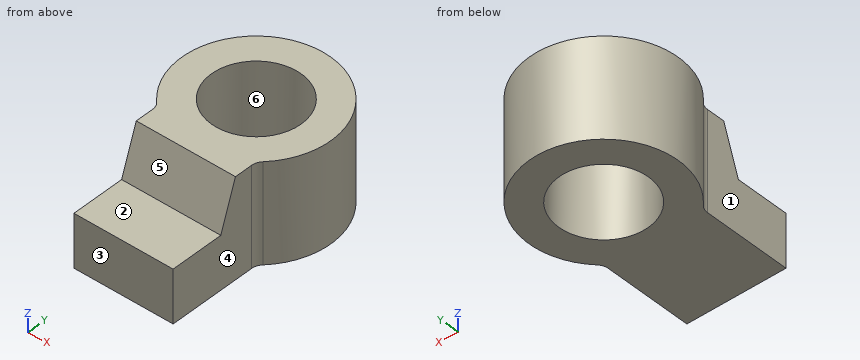
from build123d import *

# Parameters (mm, degrees)
F0_R     = 22.932499
F1_DEPTH = 50.8
F3_DEPTH = 38.1


with BuildPart() as f1:
    # F0 (on Top) → F1 (new body)
    with BuildSketch(Plane.XY):
        with BuildLine():
            ThreePointArc((25.377046, 2.454483), (25.848974, 4.856726), (27.194611, 6.901902))
            ThreePointArc((27.194611, 6.901902), (0, 71.686413), (-27.194611, 6.901902))
            ThreePointArc((-27.194611, 6.901902), (-25.848974, 4.856726), (-25.377046, 2.454483))
            Line((-25.377046, 2.454483), (-25.377046, -42.613587))
            Line((-25.377046, -42.613587), (25.377046, -42.613587))
            Line((25.377046, -42.613587), (25.377046, 2.454483))
        make_face()
        with Locations((0, 33.586413)):
            Circle(F0_R, mode=Mode.SUBTRACT)
    extrude(amount=F1_DEPTH)

    # F2 (on Right) → F3 (cut, symmetric)
    with BuildSketch(Plane.YZ):
        Polygon((-47.515366, 27.248772), (-42.938434, 27.030824), (-15.25889, 27.030824), (-4.361433, 57.761654), (-47.515366, 57.761654), align=None)
    extrude(amount=F3_DEPTH, both=True, mode=Mode.SUBTRACT)


solid = f1.part
Design review of the part built by this model. Coordinates are the model's own, in mm. Face numbers are marked on the shaded views. A direction names the side the tool comes from. Coordinates: 2 decimals unless noted, no trailing zeros. Order: outer loops, then holes, each group sorted by start corner. A loop starts at its lowest first (then second) coordinate and runs counter-clockwise, first axis right, second up. Notation, with made-up numbers: (88.5, 47.25) - (95.5, 47.25) arc R14 ccw to (95.5, 65.25) - close; hole circle Ø3 at (18.5, 30.5). An arc over 180 degrees is marked (long way). Put each result on its own line as item: value.
1) Take a section at D-D, the plane x = -21. Give the boundary of the cut face in (y, z), and give its area (3 significant figures).
Response values:
outline: (-42.61, 0) - (24.37, 0) - (24.37, 50.8) - (-6.83, 50.8) - (-15.26, 27.03) - (-42.61, 27.03) - close; (42.8, 0) - (65.38, 0) - (65.38, 50.8) - (42.8, 50.8) - close
area: 3,800 mm²
2) Take a section at A-A, the plane x = 0. Give the boundary of the cut face in (y, z), and give its area (3 significant figures).
Response values:
outline: (-42.61, 0) - (10.65, 0) - (10.65, 50.8) - (-6.83, 50.8) - (-15.26, 27.03) - (-42.61, 27.03) - close; (56.52, 0) - (71.69, 0) - (71.69, 50.8) - (56.52, 50.8) - close
area: 2,730 mm²
3) Insertion check: P1, Ø12, axis at x = 18, z = 12, coming from the +Y side; P2, Ø22, axis at x = 3, y = -33.5, coming from the +Z side; P3, Ø22.5, axis at y = -21.5, z = 30.5, coming from the +X side. Each pin has a flat end and moves straight along its axis. Give the tip position at first contact, or say it passes through.
Response values:
P1: stops at y = 69.75
P2: stops at z = 27.03
P3: stops at x = 25.38
4) Wall thickness on L1, parallel to Y at x = 0, z = 23; L2, parallel to Z at x = -25, y = -19; L3, parallel to X at y = 2.5, z = 43: over which ranges is each line inside the solid? List them lowest first. Write a range as from..to.
Response values:
L1: y = -42.61..10.65, 56.52..71.69
L2: z = 0..27.03
L3: x = -25.38..25.38
5) Take a section at B-B, the plane y = 51. Give the boundary of the cut face in (x, z), and give its area (3 significant figures).
Response values:
outline: (-33.89, 0) - (-14.92, 0) - (-14.92, 50.8) - (-33.89, 50.8) - close; (14.92, 0) - (33.89, 0) - (33.89, 50.8) - (14.92, 50.8) - close
area: 1,930 mm²
6) Tool access review of the marked faces 1, 2 and 3: name each direction out of +Z, -Z, +X, -X, +Y, -Y from which nothing blocks a thin tool from reaching the whole face with its end or side.
Response values:
face 1: +Z, -Z, -X, -Y
face 2: +Z, +X, -X, -Y
face 3: +Z, -Z, +X, -X, -Y
7) The part is to be moulded in two halves that separate along Y. For the marked faces 4, 5 and 6, say which applies: released by +Y, released by -Y, zero draft, split by the parting line, or undercut.
Response values:
face 4: zero draft
face 5: released by -Y
face 6: undercut
